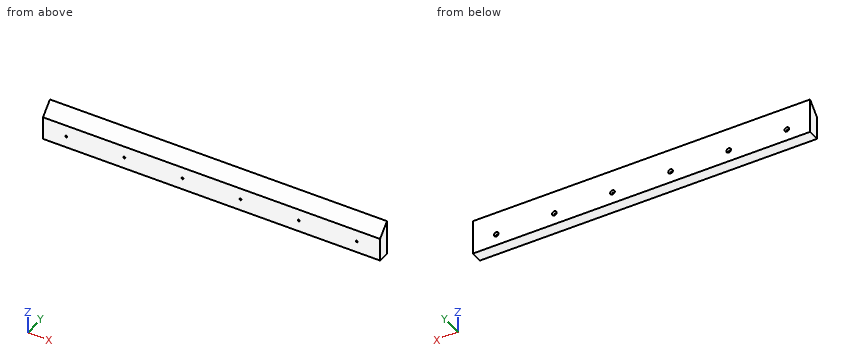
from build123d import *

# Parameters (mm, degrees)
F4_W           = 25
F4_H           = 75
F0_DEPTH       = 724
F1_SIZE        = 24.99999
F3_D           = 4
F3_CSINK_D     = 10
F3_CSINK_ANGLE = 90


# Not quite as in the source:
# - a fillet or chamfer is up to 0.001 mm smaller than in the source, because OpenCascade refuses the exact size
# - a feature names something its author has since deleted; it is built from what else it names


with BuildPart() as f0:
    # F4 (on Right) → F0 (new body)
    with BuildSketch(Plane.YZ):
        Rectangle(F4_W, F4_H)
    extrude(amount=F0_DEPTH)

    # F1 (size 25 in the source; OpenCascade refuses exactly that, so slightly less here)
    f1_edges = [f0.edges().sort_by_distance(p)[0] for p in [
        (362, -12.5, 37.5),
    ]]
    chamfer(f1_edges, length=F1_SIZE)

    # F3 (through all)
    with Locations(Plane(origin=(0, 12.5, 0), x_dir=(-1, 0, 0), z_dir=(0, 1, 0))):
        with Locations((-50, -12.5), (-174.8, -12.5), (-299.6, -12.5), (-424.4, -12.5), (-549.2, -12.5), (-674, -12.5)):
            CounterSinkHole(F3_D / 2, F3_CSINK_D / 2, counter_sink_angle=F3_CSINK_ANGLE)


solid = f0.part
Model file for the job. Use its own axes, mm. Give positions to 0.01 mm unless a question says otherwise; leave off trailing zeros. Order: outer loops, then holes, each group sorted by start corner. A loop starts at its lowest first (then second) coordinate and runs counter-clockwise, first axis right, second up. Notation, with made-up numbers: (10, -39) - (49, -39) arc R31 ccw to (49, -4) - close; hole circle Ø8 at (59, 81). An arc over 180 degrees is marked (long way). Return JSON: item names as keys, results as strings.
1) Cut at A-A, the plane y = 0.75. Give the cut face in (x, z).
Geometry says:
{"outline": "(0, -37.5) - (724, -37.5) - (724, 25.75) - (0, 25.75) - close; hole circle Ø4 at (50, -12.5); hole circle Ø4 at (174.8, -12.5); hole circle Ø4 at (299.6, -12.5); hole circle Ø4 at (424.4, -12.5); hole circle Ø4 at (549.2, -12.5); hole circle Ø4 at (674, -12.5)"}
2) Flat gauge pins, fed straight in: P1, Ø2, axis at x = 163.5, z = 20.5, coming from the -Y side; P2, Ø12, axis at x = 216, y = -7, coming from the +Z side. Where does each tip first touch, or does it go through?
Geometry says:
{"P1": "y = -5.5", "P2": "z = 24"}
3) Cut at C-C, the plane z = 24. Give the cut face in (x, y).
Geometry says:
{"outline": "(0, -1) - (724, -1) - (724, 12.5) - (0, 12.5) - close"}
4) Probe line 1 (Z direction, x = 674, y = 2); line 2 (Z direction, x = 299.6, y = -1.5); line 3 (Z direction, x = 609, y = -4.5). List the from-to ranges inside material, lowest first. Write a range as from..to.
Geometry says:
{"line 1": "-37.5..-14.5, -10.5..27", "line 2": "-37.5..-14.5, -10.5..23.5", "line 3": "-37.5..20.5"}
